Source: CAD feature listing. Evaluate the final solid. Frame: model axes, mm. A direction names the side the tool comes from. Give positions to 0.01 mm unless a question says otherwise; leave off trailing zeros. Loops run counter-clockwise (first coordinate to the right, second up) from the corner with the lowest first, then second, coordinate; pieces in that order, holes last. Notation, with made-up numbers: (21, 43) -> (51, 43) arc R7 ccw to (51, 52) -> close; hole circle Ø3 at (82, 19.5). An arc over 180 degrees is marked (long way). Put each result on its own line as item: value.
```python
from build123d import *

# Parameters (mm, degrees)
SKETCH2_R           = 2
BOSS_EXTRUDE1_DEPTH = 10
CHAMFER1_SIZE       = 0.525
CUT_EXTRUDE1_DEPTH  = 2.42


with BuildPart() as part:
    # Sketch2 → Boss-Extrude1 (new body)
    with BuildSketch(Plane(origin=(5, 0, 0), x_dir=(0, 0, -1), z_dir=(1, 0, 0))):
        Circle(SKETCH2_R)
    extrude(amount=-BOSS_EXTRUDE1_DEPTH)

    # Chamfer1
    chamfer1_edges = [part.edges().sort_by_distance(p)[0] for p in [
        (5, 0, 2),
    ]]
    chamfer(chamfer1_edges, length=CHAMFER1_SIZE)

    # Sketch6 → Revolve1 (revolve)
    with BuildSketch(Plane.XY):
        Polygon((-7.45, 3.5), (-7.8, 3.15), (-7.8, 0), (-5, 0), (-5, 3.5), align=None)
    revolve(axis=Axis((-5, 0, 0), (-1, 0, 0)))

    # Sketch4 → Cut-Extrude1 (cut)
    with BuildSketch(Plane(origin=(-7.8, 0, 0), x_dir=(0, 0, -1), z_dir=(1, 0, 0))):
        Polygon((0, 1.443375673), (-1.25, 0.721687836), (-1.25, -0.721687836), (0, -1.443375673), (1.25, -0.721687836), (1.25, 0.721687836), align=None)
    extrude(amount=CUT_EXTRUDE1_DEPTH, mode=Mode.SUBTRACT)

    # Cut-Extrude2 cone 1 section (through the dimple's axis) → Cut-Extrude2 (revolve, cut)
    with BuildSketch(Plane(origin=(-7.8, 0, 0), x_dir=(0, 0, 1), z_dir=(0, 1, 0))):
        Polygon((0, 0), (1.443375673, 0), (0, 1.443375673), align=None)
    revolve(axis=Axis((-7.8, 0, 0), (1, 0, 0)), mode=Mode.SUBTRACT)


solid = part.part
```
(1) First-contact query: P1, Ø3, axis at y = 0.5, z = 0.5, coming from the -X side; P2, Ø2, axis at x = -4.5, y = -1.5, coming from the +Z side. Flat tips, straight axial feed; report the tip coordinate or a pass-through.
Calculated:
P1: stops at x = -7.8
P2: stops at z = 3.44
(2) Line query: probe 1 along X at (y, z) = (0.5, 3); probe 2 along X at (y, z) = (-0.75, 0.5); probe 3 along Y at (x, z) = (-2, -1). Output: solid intervals per line, ascending. Write a range as from..to.
Calculated:
probe 1: x = -7.8..-5
probe 2: x = -5.38..5
probe 3: y = -1.73..1.73
(3) Reachability of faces 1 (the flat face through (-6.607, 1.088, 0.616)), 2 (the flat face through (5, 0, 0)), 3 (the cylindrical face through (0, -2, 0)) from +Z, -Z, +X, -X, +Y, -Y: full face, straight path, thin tool, end or side. Return the list, or none.
Calculated:
face 1: -X
face 2: +Z, -Z, +X, +Y, -Y
face 3: +X
(4) Draft query along Z for faces 4 (the flat face through (-7, 0, 1.25)), 5 (the cylindrical face through (-6.242, 3.233, 1.341)), 6 (the flat face through (-5, -2, 2)). Return one class per face: released by +Z, released by -Z, zero draft, split by the parting line, or undercut.
Calculated:
face 4: undercut
face 5: split by the parting line
face 6: zero draft
(5) Section A-A on x = -5.75. Return loops of the section in (y, z).
Calculated:
outline: circle Ø7 at (0, 0); hole (-1.44, 0) -> (-0.72, -1.25) -> (0.72, -1.25) -> (1.44, 0) -> (0.72, 1.25) -> (-0.72, 1.25) -> close
(6) Section B-B on y = 0. Return loops of the section in (x, z) (3 decimals), then the cut area to 3 significant figures.
Calculated:
outline: (-7.8, -3.15) -> (-7.45, -3.5) -> (-5, -3.5) -> (-5, -2) -> (4.475, -2) -> (5, -1.475) -> (5, 1.475) -> (4.475, 2) -> (-5, 2) -> (-5, 3.5) -> (-7.45, 3.5) -> (-7.8, 3.15) -> (-7.8, 1.443) -> (-7.607, 1.25) -> (-5.38, 1.25) -> (-5.38, -1.25) -> (-7.607, -1.25) -> (-7.8, -1.443) -> close
area: 53.1 mm²
(7) Section C-C on x = 1. Return loops of the section in (y, z), then the cut area to 3 significant figures.
Calculated:
outline: circle Ø4 at (0, 0)
area: 12.6 mm²
